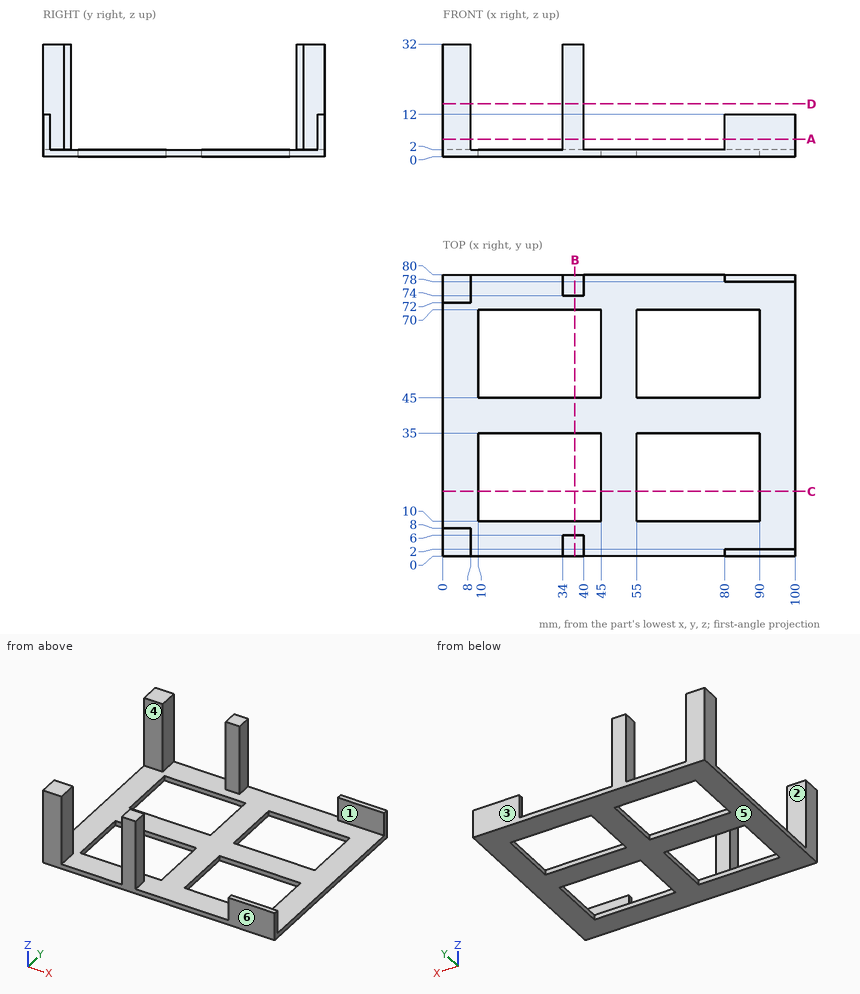
Check sheet for the drawn part. Datum: minimum x, y, z corner. Units: mm. A direction names the side the tool comes from. Coordinates: 2 decimals unless noted, no trailing zeros. Loops run counter-clockwise (first coordinate to the right, second up) from the corner with the lowest first, then second, coordinate; pieces in that order, holes last. Notation, with made-up numbers: (68, 51.25) -> (99, 51.25) arc R26 cw to (99, 88.25) -> close; hole circle Ø9 at (8.5, 25). An arc over 180 degrees is marked (long way). Answer as CSV lines item,"result".
1) Thickness scan on L1, parallel to Y at x = 94, z = 5.5; L2, parallel to Z at x = 91, y = 4; L3, parallel to Y at x = 5.5, z = 22.5. Record the ranges inside material, lowest first. Write a range as from..to.
Found:
L1,"y = 0..2, 78..80"
L2,"z = 0..2"
L3,"y = 0..8, 72..80"
2) Depth check by flat-ended pin: pin 1 (1 mm diameter, centred on x = 86, y = 1.5, fed in from +Z). Enter the tip coordinate at first touch or a pass-through.
Found:
pin 1,"stops at z = 12"
3) Cross-section at A-A, the plane z = 5. Record the cut outline in (x, y), then the cut area to 3 significant figures.
Found:
outline,"(0, 0) -> (8, 0) -> (8, 8) -> (0, 8) -> close; (0, 72) -> (8, 72) -> (8, 80) -> (0, 80) -> close; (34, 0) -> (40, 0) -> (40, 6) -> (34, 6) -> close; (34, 74) -> (40, 74) -> (40, 80) -> (34, 80) -> close; (80, 0) -> (100, 0) -> (100, 2) -> (80, 2) -> close; (80, 78) -> (100, 78) -> (100, 80) -> (80, 80) -> close"
area,"280 mm2"
4) Cross-section at D-D, the plane z = 15. Record the cut outline in (x, y), then the cut area to 3 significant figures.
Found:
outline,"(0, 0) -> (8, 0) -> (8, 8) -> (0, 8) -> close; (0, 72) -> (8, 72) -> (8, 80) -> (0, 80) -> close; (34, 0) -> (40, 0) -> (40, 6) -> (34, 6) -> close; (34, 74) -> (40, 74) -> (40, 80) -> (34, 80) -> close"
area,"200 mm2"
5) Cross-section at B-B, the plane x = 37.5. Record the cut outline in (y, z).
Found:
outline,"(0, 0) -> (10, 0) -> (10, 2) -> (6, 2) -> (6, 32) -> (0, 32) -> close; (35, 0) -> (45, 0) -> (45, 2) -> (35, 2) -> close; (70, 0) -> (80, 0) -> (80, 32) -> (74, 32) -> (74, 2) -> (70, 2) -> close"
6) Cross-section at C-C, the plane y = 18.5. Record the cut outline in (x, z), then the cut area to 3 significant figures.
Found:
outline,"(0, 0) -> (10, 0) -> (10, 2) -> (0, 2) -> close; (45, 0) -> (55, 0) -> (55, 2) -> (45, 2) -> close; (90, 0) -> (100, 0) -> (100, 2) -> (90, 2) -> close"
area,"60.0 mm2"
7) Tool access check on the marked faces 1 and 2. Record the directions out of +Z, -Z, +X, -X, +Y, -Y that give a thin tool (end or side, any length) a straight path to the whole face; none if there is none.
Found:
face 1,"+Z, +X"
face 2,"+Z, +X, -X"
8) Release check for a two-part mould opening along Y. For the marked faces 3, 4, 5 and 6 record: +Y half, -Y half, draft (parallel to the pull), parting line (faces both ways), or undercut.
Found:
face 3,"+Y half"
face 4,"undercut"
face 5,"draft"
face 6,"-Y half"
